Geometry check sheet. Reference: the model listing, model coordinates, mm. A direction names the side the tool comes from. Coordinates: 2 decimals unless noted, no trailing zeros. Order: outer loops, then holes, each group sorted by start corner. A loop starts at its lowest first (then second) coordinate and runs counter-clockwise, first axis right, second up. Notation, with made-up numbers: M -17.5,-39 L 6.5,-39 A18 cw 6.5,-30 Z; hole C -2.75,62.25 d1. An arc over 180 degrees is marked long. One line per item, written item: value. Start each with the question number.
1) Access from +Z, -Z, +X, -X, +Y, -Y to the whole of each face (thin tool, end or side, straight path). Record for faces 4 (the flat face through (13, -33.02, -5)), 5 (the cylindrical face through (-14.5, 18.3, 2.6)), 6 (the flat face through (-6.985, -31, 2)), 7 (the flat face through (-6.985, 0, 3)).
2) Thickness scan on L1, parallel to Y at x = 0, z = 1; L2, parallel to X at y = -6, z = 2.5 (3 decimals); L3, parallel to Z at x = -6.5, y = 15. Record the ranges inside material, lowest first. Write a range as from..to.
3) Sectioned sample at A-A, the plane x = -2. Enter the section's corners in (y, z).
4) Sectioned sample at C-C, the plane y = -34. Enter the section's corners in (x, z) (1 decimal), then the cut area to 3 significant figures.
5) Draft check along Y on faces 1 (the flat face through (0, 11.43, 3)), 2 (the flat face through (11, -38.1, -2)), 3 (the cylindrical face through (-12.532, -35.524, -3.707)). Enter one of: pulls with the +Y half, pulls with the -Y half, needs draft (parallel to the pull), parting line crosses it, or undercut.
6) Sectioned sample at B-B, the plane y = -25.5. Enter the section's corners in (x, z) (3 decimals).
7) Go/stop test with flat-tipped pins: P1, Ø2, axis at x = 2.5, z = -0.5, coming from the -Y side; P2, Ø1.9, axis at x = -11.11, z = -4.44, coming from the +Y side; P3, Ø4, axis at x = -10, z = -4.5, coming from the +Y side. Record where each tip stops, or that it passes through.
8) Sectioned sample at D-D, the plane z = 3. Enter the section's corners in (x, y) (3 decimals), then the cut area to 3 significant figures.
```python
from build123d import *

# Parameters (mm, degrees)
SKETCH1_W           = 8.255
SKETCH1_H           = 19.05
SKETCH1_W_2         = 13.97
SKETCH1_H_2         = 22.86
BOSS_EXTRUDE1_DEPTH = 5.08
FILLET1_R           = 2.54
SKETCH3_W           = 8.255
SKETCH3_H           = 8.89
BOSS_EXTRUDE2_DEPTH = 5.08
SKETCH5_R           = 1.016
CUT_EXTRUDE1_DEPTH  = 5.08
SKETCH6_R           = 1.6
CUT_EXTRUDE2_DEPTH  = 5.08
FILLET2_R           = 1.27
SKETCH7_W           = 4
SKETCH7_H           = 3
CUT_EXTRUDE3_DEPTH  = 44.347762341


with BuildPart() as part:
    # Sketch1 → Boss-Extrude1 (new body)
    # profile 1 of 3: a face of its own
    with BuildSketch(Plane.XY):
        with Locations((-11.1125, -28.575)):
            Rectangle(SKETCH1_W, SKETCH1_H)
    # profile 2 of 3: a face of its own
    with BuildSketch(Plane.XY):
        Polygon((-15.24, 19.05), (-15.24, -19.05), (-6.985, -19.05), (6.985, -19.05), (15.24, -19.05), (15.24, 19.05), align=None)
        Rectangle(SKETCH1_W_2, SKETCH1_H_2, mode=Mode.SUBTRACT)
    # profile 3 of 3: a face of its own
    with BuildSketch(Plane.XY):
        with Locations((11.1125, -28.575)):
            Rectangle(SKETCH1_W, SKETCH1_H)
    extrude(amount=BOSS_EXTRUDE1_DEPTH)

    # Fillet1
    fillet1_edges = [part.edges().sort_by_distance(p)[0] for p in [
        (-15.24, 19.05, 2.54),
        (15.24, 19.05, 2.54),
    ]]
    fillet(fillet1_edges, radius=FILLET1_R)

    # Sketch3 → Boss-Extrude2 (add)
    with BuildSketch(Plane(origin=(0, -38.1, 0), x_dir=(1, 0, 0), z_dir=(0, 1, 0))):
        with Locations((-11.1125, 4.445)):
            Rectangle(SKETCH3_W, SKETCH3_H)
    boss_extrude2 = extrude(amount=BOSS_EXTRUDE2_DEPTH)

    # Sketch5 → Cut-Extrude1 (cut)
    with BuildSketch(Plane.XY.offset(5.08)):
        with Locations((0, 13.97)):
            Circle(SKETCH5_R)
        with Locations((0, -13.716)):
            Circle(SKETCH5_R)
    extrude(amount=-CUT_EXTRUDE1_DEPTH, mode=Mode.SUBTRACT)

    # Sketch6 → Cut-Extrude2 (cut)
    with BuildSketch(Plane(origin=(0, -33.02, 0), x_dir=(1, 0, 0), z_dir=(0, 1, 0))):
        with Locations(Location((-11.1125, 4.445, 0), (0, 0, 270))):
            Circle(SKETCH6_R)
    cut_extrude2 = extrude(amount=-CUT_EXTRUDE2_DEPTH, mode=Mode.SUBTRACT)

    # Mirror2: Boss-Extrude2, Cut-Extrude2 across plane
    add(boss_extrude2.mirror(Plane(origin=(0, 0, 0), x_dir=(0, 0, 1), z_dir=(1, 0, 0))))
    add(cut_extrude2.mirror(Plane(origin=(0, 0, 0), x_dir=(0, 0, 1), z_dir=(1, 0, 0))), mode=Mode.SUBTRACT)

    # Fillet2
    fillet2_edges = [part.edges().sort_by_distance(p)[0] for p in [
        (15.24, -35.56, -8.89),
        (6.985, -35.56, -8.89),
        (-6.985, -35.56, -8.89),
        (-15.24, -35.56, -8.89),
    ]]
    fillet(fillet2_edges, radius=FILLET2_R)

    # Sketch7 → Cut-Extrude3 (cut, through all)
    with BuildSketch(Plane.XY.offset(5.08)):
        with Locations((4.985, -12.93)):
            Rectangle(SKETCH7_W, SKETCH7_H)
    extrude(amount=-CUT_EXTRUDE3_DEPTH, mode=Mode.SUBTRACT)


solid = part.part
```
Final values:
1. face 4: -Z, +X, -X, +Y
1. face 5: +Z, -Z, -X, +Y
1. face 6: +Z, -Z, -Y
1. face 7: +Z, -Z
2. L1: y = -19.05..-14.73, -12.7..-11.43, 11.43..12.95, 14.99..19.05
2. L2: x = -15.24..-6.985, 6.985..15.24
2. L3: z = 0..5.08
3. outline: M -19.05,0 L -11.43,0 L -11.43,5.08 L -19.05,5.08 Z; M 11.43,0 L 19.05,0 L 19.05,5.08 L 11.43,5.08 Z
4. outline: M -15.2,-7.6 A1.3 ccw -14,-8.9 L -8.3,-8.9 A1.3 ccw -7,-7.6 L -7,5.1 L -15.2,5.1 Z; M 7,-7.6 A1.3 ccw 8.3,-8.9 L 14,-8.9 A1.3 ccw 15.2,-7.6 L 15.2,5.1 L 7,5.1 Z; hole C -11.1,-4.4 d3.2; hole C 11.1,-4.4 d3.2
4. area: 213 mm^2
5. face 1: undercut
5. face 2: pulls with the -Y half
5. face 3: needs draft
6. outline: M -15.24,0 L -6.985,0 L -6.985,5.08 L -15.24,5.08 Z; M 6.985,0 L 15.24,0 L 15.24,5.08 L 6.985,5.08 Z
7. P1: stops at y = -19.05
7. P2: passes through
7. P3: stops at y = -33.02
8. outline: M -15.24,-38.1 L -6.985,-38.1 L -6.985,-19.05 L 6.985,-19.05 L 6.985,-38.1 L 15.24,-38.1 L 15.24,16.51 A2.54 ccw 12.7,19.05 L -12.7,19.05 A2.54 ccw -15.24,16.51 Z; hole M -6.985,-11.43 L 2.985,-11.43 L 2.985,-14.43 L 6.985,-14.43 L 6.985,11.43 L -6.985,11.43 Z; hole C 0,-13.716 d2.032; hole C 0,13.97 d2.032
8. area: 1,140 mm^2
